Autodesk Inventor part; units mm, degrees
ref_plane "Work Plane1" through (6.4921, 0, 2.8) normal (0, -0.9962, -0.0872) x (-1, 0, 0)
ref_plane "Work Plane2" through (6.4921, 0, 2.8) normal (0, -0.9962, 0.0872) x (-1, 0, 0)
ref_plane "YZ Plane" through (0, 0, 0) normal (1, 0, 0) x (0, 1, 0)
sketch "Sketch1" plane through (0, 0, 0) normal (0, 0, 1) x (1, 0, 0)
  circle A0 centre (0, 0) radius 2
  dimension "d0" = 4
extrude "Extrusion1" add sketch "Sketch1" along normal blind 38
ref_plane "Work Plane1" through (6.4921, 0, 2.8) normal (0, -0.9962, -0.0872) x (-1, 0, 0)
sketch "Sketch3" plane through (6.4921, 0, 2.8) normal (0, -0.9962, -0.0872) x (-1, 0, 0)
  ellipse E0 centre (6.4921, 0) end of major axis (6.4921, -22.9474) minor radius 2 (4.5072, 2.8107) -> (8.477, 2.8107) ccw
  line L0 (4.5072, 2.8107) -> (8.477, 2.8107)
  ellipse E1 centre (6.4921, 2.7893) end of major axis (8.4921, 2.7893) minor radius 0.1743
  circle A0 centre (6.4921, 0) radius 1
  point P0 (6.4921, -0.0107)
  dimension "d6" = 2.8
  dimension "d14" = 2
extrude "Extrusion2" cut sketch "Sketch3" along normal through all both and the other way through all contours A0
ref_plane "Work Plane2" through (6.4921, 0, 2.8) normal (0, -0.9962, 0.0872) x (-1, 0, 0)
sketch "Sketch5" plane through (6.4921, 0, 2.8) normal (0, -0.9962, 0.0872) x (-1, 0, 0)
  circle A0 centre (6.4921, 0.0156) radius 1
  point P0 (6.4921, 2.7893)
  dimension "d18" = 2
extrude "Extrusion3" cut sketch "Sketch5" along normal through all both and the other way through all
sketch "Sketch7" plane through (0, 0, 38) normal (0, 0, 1) x (1, 0, 0)
  circle A0 centre (0, 0) radius 2
  circle A1 centre (0, 0) radius 1.8
  dimension "d27" = 3.6
extrude "Extrusion4" cut sketch "Sketch7" against normal blind 6
chamfer "Chamfer2" distance 0.25 angle 45 2 edges at (-1.8, 0, 38) (-2, 0, 0)
properties part number "Link Arm1"
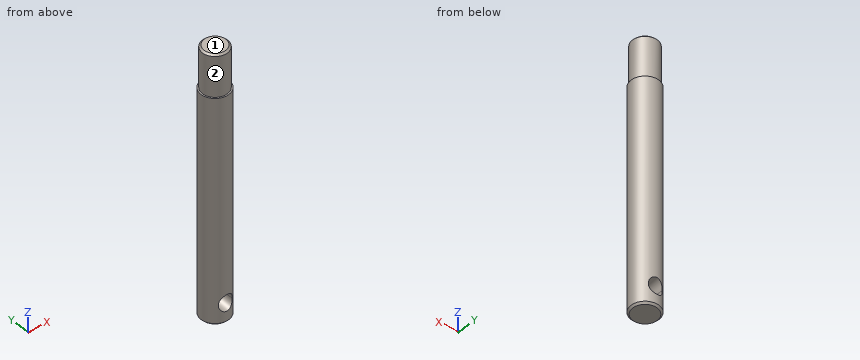
The model under review builds one solid part; all positions refer to its coordinate system, in mm. Face numbers are marked on the shaded views. A direction names the side the tool comes from. Round coordinates to 2 decimals unless told otherwise and drop trailing zeros. Write each loop counter-clockwise with the first axis right and the second up, starting at its lowest first coordinate (ties: lowest second). Pieces come first, ordered by that corner, then holes. Notation, with made-up numbers: M -38,53 L -2,53 A26 ccw -2,92 Z; hole C 21.5,-26 d5. An arc over 180 degrees is marked long. Use a Markdown table: item, result. Add a question column.
Q1. To check wall thickness, follow line 1 (Z direction, x = -0.75, y = -0.85); line 2 (X direction, y = -1.25, z = 2); line 3 (Z direction, x = -0.65, y = -0.15). State the ranges of each line that lie inside material, in increasing order.
Q2. Insertion check: pin 1 (1 mm diameter, centred on x = 0.5, z = 18, fed in from -Y); pin 2 (1 mm diameter, centred on x = -1, z = 32, fed in from -Y); pin 3 (1 mm diameter, centred on y = -1, z = 6, fed in from -X). Each pin has a flat end and moves straight along its axis. Give the tip position at first contact, or say it passes through.
Q3. Machinability: for the marked faces 1 and 2, which of the approach directions +Z, -Z, +X, -X, +Y, -Y give a long, thin tool a straight path to every point of the face, cutting with its end or side? Answer none if there is none.
Q4. We need section A-A, the plane x = 0. State the section outline as (y, z) points, plus the area to 3 significant figures.
Q5. We need section B-B, the plane z = 14. State the section outline as (x, y) points, plus the area to 3 significant figures.
Findings below:
| question | item | result |
|---|---|---|
| 1 | line 1 | z = 0 to 2.06, 3.52 to 38 |
| 1 | line 2 | x = -1.56 to -0.73, 0.73 to 1.56 |
| 1 | line 3 | z = 0 to 2.02, 3.56 to 38 |
| 2 | pin 1 | stops at y = -2 |
| 2 | pin 2 | stops at y = -1.94 |
| 2 | pin 3 | stops at x = -1.94 |
| 3 | face 1 | +Z, +X, -X, +Y, -Y |
| 3 | face 2 | +Z |
| 4 | outline | M -2,0.25 L -1.75,0 L 1.75,0 L 2,0.25 L 2,1.61 L -0.09,1.79 L -2,1.62 Z; M -2,3.96 L -0.09,3.8 L 2,3.98 L 2,32 L 1.8,32 L 1.8,37.75 L 1.55,38 L -1.55,38 L -1.8,37.75 L -1.8,32 L -2,32 Z |
| 4 | area | 141 mm² |
| 5 | outline | C 0,0 d4 |
| 5 | area | 12.6 mm² |
